Source: CAD feature listing. Evaluate the final solid. Frame: model axes, mm. A direction names the side the tool comes from. Round coordinates to 2 decimals unless told otherwise and drop trailing zeros. Loops run counter-clockwise (first coordinate to the right, second up) from the corner with the lowest first, then second, coordinate; pieces in that order, holes last. Notation, with made-up numbers: M 58,-32 L 83,-32 A23 ccw 83,-24 Z; hole C -11.75,86 d6. An arc over 180 degrees is marked long. Answer as a JSON object with one key per item and string values.
from build123d import *

# Parameters (mm, degrees)
EXTRUDE008_DEPTH = 2


with BuildPart() as obj1:
    # Sketch011 → Revolve (revolve)
    with BuildSketch(Plane.YZ):
        Polygon((43.6433333333, 6.6666666667), (43.6433333333, 7.3333333333), (44.31, 8), (44.31, 14), (40, 14), (40, 6), (44.31, 6), align=None)
    revolve(axis=Axis((0, 40, 6), (0, 0, -1)))


with BuildPart() as obj2:
    # Sketch009 (on Face8 of Extrude003) → Extrude008 (new body)
    with BuildSketch(Plane.XY.offset(6)):
        with BuildLine():
            Line((-8.62, 40), (-8.62, 18.3899891245))
            ThreePointArc((-8.62, 18.3899891245), (0, -20.31), (8.62, 18.3899891245))
            Line((8.62, 40), (8.62, 18.3899891245))
            ThreePointArc((8.62, 40), (0, 48.62), (-8.62, 40))
        make_face()
        with BuildLine():
            Line((-4.62, 16.31), (4.62, 16.31))
            Line((4.62, 7.2773621595), (4.62, 16.31))
            ThreePointArc((4.62, -7.2773621595), (8.62, 0), (4.62, 7.2773621595))
            Line((4.62, -7.2773621595), (4.62, -16.31))
            Line((4.62, -16.31), (-4.62, -16.31))
            Line((-4.62, -7.2773621595), (-4.62, -16.31))
            ThreePointArc((-4.62, 7.2773621595), (-8.62, 0), (-4.62, -7.2773621595))
            Line((-4.62, 16.31), (-4.62, 7.2773621595))
        make_face(mode=Mode.SUBTRACT)
    extrude(amount=EXTRUDE008_DEPTH)

    # Cut002: cut obj1
    add(obj1.part, mode=Mode.SUBTRACT)


solid = obj2.part
Item 1: Section C-C on x = 5.5. Return the cut outline in (y, z), then the cut area to 3 significant figures.
Answer sheet:
{"outline": "M -19.55,6 L -6.64,6 L -6.64,8 L -19.55,8 Z; M 6.64,6 L 46.64,6 L 46.64,8 L 6.64,8 Z", "area": "106 mm²"}
Item 2: Line query: probe 1 along X at (y, z) = (40, 7); probe 2 along Y at (x, z) = (1, 7.95); probe 3 along X at (y, z) = (42.5, 6.7). Output: solid intervals per line, ascending. Write a range as from..to.
Answer sheet:
{"probe 1": "x = -8.62..-3.64, 3.64..8.62", "probe 2": "y = -20.29..-16.31, 16.31..35.86, 44.14..48.56", "probe 3": "x = -8.25..-2.65, 2.65..8.25"}
Item 3: Section D-D on x = 10. Return the cut outline in (y, z), then the cut area to 3 significant figures.
Answer sheet:
{"outline": "M -17.68,6 L 17.68,6 L 17.68,8 L -17.68,8 Z", "area": "70.7 mm²"}
Item 4: Section A-A on x = 0. Return the cut outline in (y, z).
Answer sheet:
{"outline": "M -20.31,6 L -16.31,6 L -16.31,8 L -20.31,8 Z; M 16.31,6 L 35.69,6 L 36.36,6.67 L 36.36,7.33 L 35.69,8 L 16.31,8 Z; M 43.64,6.67 L 44.31,6 L 48.62,6 L 48.62,8 L 44.31,8 L 43.64,7.33 Z"}
Item 5: Contact query for flat-ended pins moving along their axis: pin 1 Ø1 at (y, z) = (24, 7.5) entering from -X; pin 2 Ø6.5 at (x, y) = (0, 40) entering from -Z; pin 3 Ø0.6 at (y, z) = (-12, 7) entering from -X; pin 4 Ø0.6 at (x, z) = (-1.5, 7) entering from -Y. Output: stop coordinate, or through.
Answer sheet:
{"pin 1": "stops at x = -8.62", "pin 2": "passes through", "pin 3": "stops at x = -16.6", "pin 4": "stops at y = -20.27"}
Item 6: Section B-B on y = 0. Return the cut outline in (x, z), then the cut area to 3 significant figures.
Answer sheet:
{"outline": "M -20.31,6 L -8.62,6 L -8.62,8 L -20.31,8 Z; M 8.62,6 L 20.31,6 L 20.31,8 L 8.62,8 Z", "area": "46.8 mm²"}
Item 7: Access query for faces 1 (the flat face through (-8.62, 29, 7)), 2 (the flat face through (4.62, 12, 7)), 3 (the flat face through (-5, 15, 8)), 4 (the flat face through (8.62, 29, 7)). Directions: +Z, -Z, +X, -X, +Y, -Y. A direction counts if a zero-diameter tool reaches every point of the face in a straight line with its end or side. Return the directions, or none.
Answer sheet:
{"face 1": "+Z, -Z, -X, +Y", "face 2": "+Z, -Z", "face 3": "+Z, +X, -X, +Y, -Y", "face 4": "+Z, -Z, +X, +Y"}
Item 8: Pull-direction query (Y, two-part tool) for faces 5 (the flat face through (0, 16.31, 7)), 6 (the flat face through (-4.62, 12, 7)), 7 (the cylindrical face through (0.19, 48.618, 6.986)), 8 (the flat face through (-5, 15, 6)); classes: pulls with the +Y half, pulls with the -Y half, needs draft (parallel to the pull), parting line crosses it, or undercut.
Answer sheet:
{"face 5": "undercut", "face 6": "undercut", "face 7": "pulls with the +Y half", "face 8": "needs draft"}
